Can you work these out from the model? Positions are in its coordinate system, mm. A direction names the side the tool comes from. Coordinates: 2 decimals unless noted, no trailing zeros. Loops run counter-clockwise (first coordinate to the right, second up) from the corner with the lowest first, then second, coordinate; pieces in that order, holes last. Notation, with made-up numbers: M 23.25,-9.5 L 52.25,-9.5 A26 cw 52.25,7.5 Z; hole C -21.5,3 d3. An arc over 180 degrees is marked long. Answer as a JSON object with one key per item and string values. Group by question number.
Item 1: Suppose I cut it at A-A (z = 0). Write out the boundary of the cut face in (x, y).
Item 2: Suppose I cut it at B-B (y = 35). Write out the boundary of the cut face in (x, z).
Item 3: I'm going to push flat-ended pins straight in: pin 1 Ø11 at (x, z) = (0, -141.83) entering from +Y; pin 2 Ø3 at (x, z) = (-100, -52.5) entering from +Y. Where does each tip first touch, or does it pass through?
Item 4: Which directions (+Z, -Z, +X, -X, +Y, -Y) give clear straight access to the entire face, cutting with the end or side of a thin tool? Please do faces 1 (the cylindrical face through (-187.256, 151.907, -0.617)), 2 (the flat face through (-3, 0, -2)), 3 (the flat face through (-3, 75, 153.4)).
Item 5: Suppose I cut it at D-D (z = 61). Write out the boundary of the cut face in (x, y).
Item 6: If I drill on line 1 (X direction, y = 151.6, z = 0); line 2 (X direction, y = 115, z = -130); line 3 (Y direction, x = 130, z = -130), over which ranges is the centre line in solid material (lowest first)?
Item 7: We'd pull the mould along X, two halves only. Please class faces 4 (the cylindrical face through (188.028, 151.907, -4.012)), 5 (the flat face through (205.2, 78, 2)), 6 (the flat face through (-205.2, 76, 2)), 7 (the cylindrical face through (4.121, 151.907, 143.393)): +X half, -X half, draft (parallel to the pull), parting line (faces both ways), or undercut.
Item 8: Suppose I cut it at C-C (x = -157). Write out the boundary of the cut face in (y, z).
```python
from build123d import *

# Parameters (mm, degrees)
SKETCH1_W           = 410.4
SKETCH1_H           = 308.8
BOSS_EXTRUDE2_DEPTH = 1
SKETCH5_W           = 410.4
SKETCH5_H           = 1
BOSS_EXTRUDE4_DEPTH = 152.4
SKETCH10_W          = 1
SKETCH10_H          = 308.8
EXTRUDE_THIN2_DEPTH = 152.4
SKETCH11_W          = 1
SKETCH11_H          = 307.8
SKETCH11_W_2        = 409.4
SKETCH11_H_2        = 1
EXTRUDE_THIN3_DEPTH = 152.4
SKETCH12_W          = 410.4
SKETCH12_H          = 1
EXTRUDE_THIN4_DEPTH = 25.4
SKETCH13_W          = 308.8
SKETCH13_H          = 1
EXTRUDE_THIN5_DEPTH = 25.4
SKETCH14_W          = 410.4
SKETCH14_H          = 1
EXTRUDE_THIN6_DEPTH = 25.4
SKETCH15_W          = 308.8
SKETCH15_H          = 1
EXTRUDE_THIN7_DEPTH = 25.4
SKETCH19_R          = 5.056095902
SKETCH19_R_2        = 4.737056414
SKETCH19_R_3        = 4.194334137
SKETCH19_R_4        = 4.887308366
CUT_EXTRUDE3_DEPTH  = 10


with BuildPart() as part:
    # Sketch1 → Boss-Extrude2 (new body)
    with BuildSketch(Plane(origin=(0, 0, 0), x_dir=(1, 0, 0), z_dir=(0, 1, 0))):
        Rectangle(SKETCH1_W, SKETCH1_H)
    extrude(amount=BOSS_EXTRUDE2_DEPTH)

    # Sketch5 → Boss-Extrude4 (add)
    with BuildSketch(Plane(origin=(0, 1, 0), x_dir=(1, 0, 0), z_dir=(0, 1, 0))):
        with Locations((0, -153.9)):
            Rectangle(SKETCH5_W, SKETCH5_H)
    extrude(amount=BOSS_EXTRUDE4_DEPTH)

    # Sketch10 → Extrude-Thin2 (add)
    with BuildSketch(Plane(origin=(0, 1, 0), x_dir=(1, 0, 0), z_dir=(0, 1, 0))):
        with Locations((-204.7, 0)):
            Rectangle(SKETCH10_W, SKETCH10_H)
    extrude(amount=EXTRUDE_THIN2_DEPTH)

    # Sketch11 → Extrude-Thin3 (add)
    with BuildSketch(Plane(origin=(0, 1, 0), x_dir=(1, 0, 0), z_dir=(0, 1, 0))):
        with Locations((204.7, 0.5)):
            Rectangle(SKETCH11_W, SKETCH11_H)
        with Locations((0.5, 153.9)):
            Rectangle(SKETCH11_W_2, SKETCH11_H_2)
    extrude(amount=EXTRUDE_THIN3_DEPTH)

    # Sketch12 → Extrude-Thin4 (add)
    with BuildSketch(Plane(origin=(0, 0, -154.4), x_dir=(-1, 0, 0), z_dir=(0, 0, -1))):
        with Locations((0, 151.9)):
            Rectangle(SKETCH12_W, SKETCH12_H)
    extrude(amount=-EXTRUDE_THIN4_DEPTH)

    # Sketch13 → Extrude-Thin5 (add)
    with BuildSketch(Plane.ZY.offset(205.2)):
        with Locations((0, 151.9)):
            Rectangle(SKETCH13_W, SKETCH13_H)
    extrude(amount=-EXTRUDE_THIN5_DEPTH)

    # Sketch14 → Extrude-Thin6 (add)
    with BuildSketch(Plane.XY.offset(154.4)):
        with Locations((0, 151.9)):
            Rectangle(SKETCH14_W, SKETCH14_H)
    extrude(amount=-EXTRUDE_THIN6_DEPTH)

    # Sketch15 → Extrude-Thin7 (add)
    with BuildSketch(Plane(origin=(205.2, 0, 0), x_dir=(0, 0, -1), z_dir=(1, 0, 0))):
        with Locations((0, 151.9)):
            Rectangle(SKETCH15_W, SKETCH15_H)
    extrude(amount=-EXTRUDE_THIN7_DEPTH)

    # Sketch19 → Cut-Extrude3 (cut)
    with BuildSketch(Plane(origin=(0, 152.4, 0), x_dir=(1, 0, 0), z_dir=(0, 1, 0))):
        with Locations(Location((191.104510435, 0, 0), (0, 0, 270))):
            Circle(SKETCH19_R)
        with Locations(Location((-191.953029846, 0, 0), (0, 0, 270))):
            Circle(SKETCH19_R_2)
        with Locations(Location((0, 141.834718346, 0), (0, 0, 270))):
            Circle(SKETCH19_R_3)
        with Locations(Location((0, -140.765526806, 0), (0, 0, 270))):
            Circle(SKETCH19_R_4)
    extrude(amount=-CUT_EXTRUDE3_DEPTH, mode=Mode.SUBTRACT)


solid = part.part
```
From the geometry:
{
 "1": {"outline": "M -205.2,0 L 205.2,0 L 205.2,153.4 L 204.2,153.4 L 204.2,152.4 L 196.16,152.4 L 196.16,151.4 L 204.2,151.4 L 204.2,1 L -204.2,1 L -204.2,151.4 L -196.69,151.4 L -196.69,152.4 L -204.2,152.4 L -204.2,153.4 L -205.2,153.4 Z; M -187.22,151.4 L -179.8,151.4 L -179.8,152.4 L -187.22,152.4 Z; M 179.8,151.4 L 186.05,151.4 L 186.05,152.4 L 179.8,152.4 Z"},
 "2": {"outline": "M -205.2,-154.4 L 205.2,-154.4 L 205.2,154.4 L -205.2,154.4 Z; hole M -204.2,-153.4 L 204.2,-153.4 L 204.2,153.4 L -204.2,153.4 Z"},
 "3": {"pin 1": "y = 152.4", "pin 2": "y = 1"},
 "4": {"face 1": "+Y", "face 2": "+Z, -Z, +X, -X, -Y", "face 3": "none"},
 "5": {"outline": "M -205.2,0 L 205.2,0 L 205.2,153.4 L 204.2,153.4 L 204.2,152.4 L 179.8,152.4 L 179.8,151.4 L 204.2,151.4 L 204.2,1 L -204.2,1 L -204.2,151.4 L -179.8,151.4 L -179.8,152.4 L -204.2,152.4 L -204.2,153.4 L -205.2,153.4 Z"},
 "6": {"line 1": "-205.2 to -196.69, -187.22 to -179.8, 179.8 to 186.05, 196.16 to 205.2", "line 2": "-205.2 to -204.2, 204.2 to 205.2", "line 3": "0 to 1, 151.4 to 152.4"},
 "7": {"face 4": "undercut", "face 5": "+X half", "face 6": "-X half", "face 7": "undercut"},
 "8": {"outline": "M 0,-154.4 L 153.4,-154.4 L 153.4,-153.4 L 152.4,-153.4 L 152.4,-129 L 151.4,-129 L 151.4,-153.4 L 1,-153.4 L 1,153.4 L 151.4,153.4 L 151.4,129 L 152.4,129 L 152.4,153.4 L 153.4,153.4 L 153.4,154.4 L 0,154.4 Z"}
}
